from build123d import *

# Parameters (mm, degrees)
SKETCH1_W               = 204.5
SKETCH1_H               = 62.5
BOSS_EXTRUDE1_DEPTH     = 3
SKETCH2_R               = 8
BOSS_EXTRUDE2_DEPTH     = 7
SKETCH3_R               = 22
BOSS_EXTRUDE3_DEPTH     = 7
SKETCH4_R               = 2.165
CUT_EXTRUDE1_DEPTH      = 108.147678463
CUT_EXTRUDE3_DEPTH      = 7
MIRROR2_COPY_1_SKETCH_R = 2.165
MIRROR2_COPY_1_DEPTH    = 108.147678463
MIRROR2_COPY_2_DEPTH    = 7
MIRROR2_COPY_3_SKETCH_R = 2.165
MIRROR2_COPY_3_DEPTH    = 108.147678463
SKETCH7_R               = 18.5
CUT_EXTRUDE4_DEPTH      = 7
SKETCH11_R              = 4
CUT_EXTRUDE7_DEPTH      = 7
SKETCH12_R              = 15
CUT_EXTRUDE8_DEPTH      = 105.82395957
SKETCH13_R              = 2.165
CUT_EXTRUDE9_DEPTH      = 105.82395957


with BuildPart() as part:
    # Sketch1 → Boss-Extrude1 (new body)
    with BuildSketch(Plane.XY):
        Rectangle(SKETCH1_W, SKETCH1_H)
    extrude(amount=BOSS_EXTRUDE1_DEPTH)

    # Sketch2 → Boss-Extrude2 (add)
    with BuildSketch(Plane.XY.offset(3)):
        with Locations(Location((-87.5, 0, 0), (0, 0, 180))):
            Circle(SKETCH2_R)
        with Locations(Location((87.5, 0, 0), (0, 0, 180))):
            Circle(SKETCH2_R)
    extrude(amount=BOSS_EXTRUDE2_DEPTH)

    # Sketch3 → Boss-Extrude3 (add)
    with BuildSketch(Plane.XY.offset(3)):
        with Locations(Location((0, 0, 0), (0, 0, 180))):
            Circle(SKETCH3_R)
    extrude(amount=BOSS_EXTRUDE3_DEPTH)

    # Sketch4 → Cut-Extrude1 (cut, through all)
    with BuildSketch(Plane.XY.offset(3)):
        with Locations((-96.5, 9)):
            Circle(SKETCH4_R)
        with Locations((-96.5, -9)):
            Circle(SKETCH4_R)
    cut_extrude1 = extrude(amount=-CUT_EXTRUDE1_DEPTH, mode=Mode.SUBTRACT)

    # Sketch6 → Cut-Extrude3 (cut)
    with BuildSketch(Plane.XY.offset(3)):
        with BuildLine():
            Line((-102.25, 0), (-102.25, -9))
            ThreePointArc((-102.25, -9), (-101.935103767, -7.123261595), (-101.024905378, -5.452080705))
            Line((-101.024905378, -5.452080705), (-96.75, 0))
            Line((-96.75, 0), (-102.25, 0))
        make_face()
        with BuildLine():
            Line((-40, -8), (-82.092970466, -8))
            ThreePointArc((-82.092970466, -8), (-87.608403359, -9.22799932), (-92.081844276, -12.68))
            ThreePointArc((-92.081844276, -12.68), (-98.456796437, -14.406796437), (-102.25, -9))
            Line((-102.25, -9), (-102.25, -31.25))
            Line((-102.25, -31.25), (0, -31.25))
            Line((0, -31.25), (0, -22))
            Line((0, -22), (-26, -22))
            Line((-26, -22), (-40, -8))
        make_face()
    cut_extrude3 = extrude(amount=-CUT_EXTRUDE3_DEPTH, mode=Mode.SUBTRACT)

    # Mirror1: Cut-Extrude1, Cut-Extrude3 across plane
    add(cut_extrude1.mirror(Plane(origin=(0, 0, 0), x_dir=(0, 0, 1), z_dir=(1, 0, 0))), mode=Mode.SUBTRACT)
    add(cut_extrude3.mirror(Plane(origin=(0, 0, 0), x_dir=(0, 0, 1), z_dir=(1, 0, 0))), mode=Mode.SUBTRACT)

    # Mirror2: Cut-Extrude3 across plane
    add(cut_extrude3.mirror(Plane.ZX), mode=Mode.SUBTRACT)

    # Mirror2 copy 1 sketch → Mirror2 copy 1 (cut, through all)
    with BuildSketch(Plane(origin=(0, 0, 3), x_dir=(-1, 0, 0), z_dir=(0, 0, 1))):
        with Locations((-96.5, 9)):
            Circle(MIRROR2_COPY_1_SKETCH_R)
        with Locations((-96.5, -9)):
            Circle(MIRROR2_COPY_1_SKETCH_R)
    extrude(amount=-MIRROR2_COPY_1_DEPTH, mode=Mode.SUBTRACT)

    # Mirror2 copy 2 sketch → Mirror2 copy 2 (cut)
    with BuildSketch(Plane(origin=(0, 0, 3), x_dir=(-1, 0, 0), z_dir=(0, 0, 1))):
        with BuildLine():
            Line((-102.25, 0), (-102.25, -9))
            ThreePointArc((-102.25, -9), (-101.935103767, -7.123261595), (-101.024905378, -5.452080705))
            Line((-101.024905378, -5.452080705), (-96.75, 0))
            Line((-96.75, 0), (-102.25, 0))
        make_face()
        with BuildLine():
            Line((-40, -8), (-82.092970466, -8))
            ThreePointArc((-82.092970466, -8), (-87.608403359, -9.22799932), (-92.081844276, -12.68))
            ThreePointArc((-92.081844276, -12.68), (-98.456796437, -14.406796437), (-102.25, -9))
            Line((-102.25, -9), (-102.25, -31.25))
            Line((-102.25, -31.25), (0, -31.25))
            Line((0, -31.25), (0, -22))
            Line((0, -22), (-26, -22))
            Line((-26, -22), (-40, -8))
        make_face()
    extrude(amount=-MIRROR2_COPY_2_DEPTH, mode=Mode.SUBTRACT)

    # Mirror2 copy 3 sketch → Mirror2 copy 3 (cut, through all)
    with BuildSketch(Plane.XY.offset(3)):
        with Locations((-96.5, -9)):
            Circle(MIRROR2_COPY_3_SKETCH_R)
        with Locations((-96.5, 9)):
            Circle(MIRROR2_COPY_3_SKETCH_R)
    extrude(amount=-MIRROR2_COPY_3_DEPTH, mode=Mode.SUBTRACT)

    # Sketch7 → Cut-Extrude4 (cut)
    with BuildSketch(Plane.XY.offset(10)):
        Circle(SKETCH7_R)
    extrude(amount=-CUT_EXTRUDE4_DEPTH, mode=Mode.SUBTRACT)

    # Sketch11 → Cut-Extrude7 (cut)
    with BuildSketch(Plane.XY.offset(10)):
        with Locations((-87.5, 0)):
            Circle(SKETCH11_R)
        with Locations((87.5, 0)):
            Circle(SKETCH11_R)
    extrude(amount=-CUT_EXTRUDE7_DEPTH, mode=Mode.SUBTRACT)

    # Sketch12 → Cut-Extrude8 (cut, through all)
    with BuildSketch(Plane.XY.offset(3)):
        Circle(SKETCH12_R)
    extrude(amount=-CUT_EXTRUDE8_DEPTH, mode=Mode.SUBTRACT)

    # Sketch13 → Cut-Extrude9 (cut, through all)
    with BuildSketch(Plane.XY.offset(3)):
        with Locations((-25, 12.5)):
            Circle(SKETCH13_R)
        with Locations((-25, -12.5)):
            Circle(SKETCH13_R)
        with Locations((25, -12.5)):
            Circle(SKETCH13_R)
        with Locations((25, 12.5)):
            Circle(SKETCH13_R)
    extrude(amount=-CUT_EXTRUDE9_DEPTH, mode=Mode.SUBTRACT)


solid = part.part
Source: CAD feature listing. Evaluate the final solid. Frame: model axes, mm. A direction names the side the tool comes from. Round coordinates to 2 decimals unless told otherwise and drop trailing zeros. Write each loop counter-clockwise with the first axis right and the second up, starting at its lowest first coordinate (ties: lowest second). Pieces come first, ordered by that corner, then holes. Notation, with made-up numbers: M 54.25,35.25 L 82.25,35.25 A14 ccw 82.25,57.25 Z; hole C 61,-9.75 d7. An arc over 180 degrees is marked long. One line per item, written item: value. Start each with the question number.
Item 1: Pin query (flat end, axial travel): pin 1 (6 mm diameter, centred on y = -4, z = 4, fed in from -X); pin 2 (13 mm diameter, centred on x = 68, y = 9.5, fed in from +Z); pin 3 (4 mm diameter, centred on y = -14, z = 2, fed in from +X); pin 4 (2.5 mm diameter, centred on x = -96.5, y = -9, fed in from +Z). Return the tip coordinate at first contact, or that it passes through.
Item 2: Ray query, L1, parallel to Y at x = -25, z = 2.15 (3 decimals); L2, parallel to Y at x = 0, z = 7.5; L3, parallel to Y at x = -87.5, z = 6.25. Return the intervals inside material, ascending. Write a range as from..to.
Item 3: Section query B-B (x = -70). Return the cut outline in (y, z).
Item 4: Section query A-A (x = -3). Return the cut outline in (y, z).
Item 5: Set-up query: faces 1 (the cylindrical face through (-87.536, -9.194, 1.521)), 2 (the flat face through (-88, 0, 3)), 3 (the flat face through (-98.917, 2.764, 1.521)). Return all of +Z, -Z, +X, -X, +Y, -Y with unobstructed straight access to the full face (end or side cutting, diameter ignored); none if empty.
Item 6: Mould query, pull axis X, two halves, no side actions, for faces 4 (the flat face through (-33, -15, 2)), 5 (the flat face through (98.917, 2.764, 1.521)), 6 (the flat face through (86, -4, 10)). Classes: pulls with the +X half, pulls with the -X half, needs draft (parallel to the pull), parting line crosses it, or undercut.
Result set:
1. pin 1: stops at x = -101.82
1. pin 2: stops at z = 3
1. pin 3: stops at x = 101.41
1. pin 4: passes through
2. L1: y = -22..-14.665, -10.335..10.335, 14.665..22
2. L2: y = -22..-18.5, 18.5..22
2. L3: y = -8..-4, 4..8
3. outline: M -8,0 L 8,0 L 8,3 L -8,3 Z
4. outline: M -22,0 L -14.7,0 L -14.7,3 L -18.26,3 L -18.26,10 L -21.79,10 L -21.79,3 L -22,3 Z; M 14.7,0 L 22,0 L 22,3 L 21.79,3 L 21.79,10 L 18.26,10 L 18.26,3 L 14.7,3 Z
5. face 1: +Z, -Z, -Y
5. face 2: +Z
5. face 3: +Z, -Z, -X
6. face 4: undercut
6. face 5: pulls with the +X half
6. face 6: needs draft
